```python
from build123d import *

# Parameters (mm, degrees)
SKETCH_R  = 0.95
PAD_DEPTH = 3


with BuildPart() as part:
    # Sketch → Pad (new body)
    with BuildSketch(Plane.XY):
        with BuildLine():
            ThreePointArc((1.04259, -1.342761), (1.608212, 0.551048), (0, 1.7))
            ThreePointArc((-0.965474, 1.868515), (-0.490035, 1.742445), (0, 1.7))
            Line((-5.775897, 3.600518), (-0.965474, 1.868515))
            ThreePointArc((-5.2, 6.9), (-6.874682, 5.492302), (-5.775897, 3.600518))
            Line((5.2, 6.9), (-5.2, 6.9))
            ThreePointArc((6.9, 5.2), (6.402082, 6.402082), (5.2, 6.9))
            Line((6.9, 0.351015), (6.9, 5.2))
            ThreePointArc((5.345348, -1.342761), (6.452416, -0.798531), (6.9, 0.351015))
            Line((1.182348, -1.7), (5.345348, -1.342761))
            ThreePointArc((1.04259, -1.342761), (0.978994, -1.573598), (1.182348, -1.7))
        make_face()
        with Locations((0, 5.5)):
            Circle(SKETCH_R, mode=Mode.SUBTRACT)
    extrude(amount=PAD_DEPTH)


solid = part.part
```
CAD build for the part. Positions are in the model's coordinates, mm. Coordinates: 2 decimals unless noted, no trailing zeros. Order: outer loops, then holes, each group sorted by start corner. A loop starts at its lowest first (then second) coordinate and runs counter-clockwise, first axis right, second up. Notation, with made-up numbers: (9, 36.5) - (47, 36.5) arc R17 cw to (47, 55.5) - close; hole circle Ø6 at (9, -29.75). An arc over 180 degrees is marked (long way). Answer in a Markdown table with one row per item.
1. Slice it at A-A, the plane x = 1.5. List the corners of the cut face in (y, z), then the cut area to 3 significant figures.
Answer:
| item | result |
|---|---|
| outline | (-1.67, 0) - (-0.8, 0) - (-0.8, 3) - (-1.67, 3) - close; (0.8, 0) - (6.9, 0) - (6.9, 3) - (0.8, 3) - close |
| area | 20.9 mm² |
2. Drill centre lines: L1, parallel to X at y = 6, z = 0.4; L2, parallel to Y at x = 0.5, z = 1.15; L3, parallel to X at y = 4.5, z = 1.65. Where is each one in solid material? Low to high. Write a range as from..to.
Answer:
| item | result |
|---|---|
| L1 | -6.7..-0.81, 0.81..6.7 |
| L2 | 1.62..4.69, 6.31..6.9 |
| L3 | -6.75..6.9 |
3. Pull direction X, two halves, no side cores. Call faces 1 (the face through (-0.7, 6.14, 1.48)), 2 (the face through (-6.869, 5.525, 1.479)), 3 (the face through (6.9, 3, 1)): +X half, -X half, draft (parallel to the pull), parting line (faces both ways), or undercut.
Answer:
| item | result |
|---|---|
| face 1 | undercut |
| face 2 | -X half |
| face 3 | +X half |
4. Slice it at D-D, the plane x = 5.75. List the corners of the cut face in (y, z), then the cut area to 3 significant figures.
Answer:
| item | result |
|---|---|
| outline | (-1.26, 0) - (6.81, 0) - (6.81, 3) - (-1.26, 3) - close |
| area | 24.2 mm² |
5. Slice it at C-C, the plane z = 0.45. List the corners of the cut face in (x, y), then the cut area to 3 significant figures.
Answer:
| item | result |
|---|---|
| outline | (-5.78, 3.6) - (-0.97, 1.87) arc R2.85 ccw to (0, 1.7) arc R1.7 cw to (1.04, -1.34) arc R0.2 ccw to (1.18, -1.7) - (5.35, -1.34) arc R1.7 ccw to (6.9, 0.35) - (6.9, 5.2) arc R1.7 ccw to (5.2, 6.9) - (-5.2, 6.9) arc R1.7 ccw to start; hole circle Ø1.9 at (0, 5.5) |
| area | 76.9 mm² |
6. Slice it at B-B, the plane y = 5.5. List the corners of the cut face in (x, z), then the cut area to 3 significant figures.
Answer:
| item | result |
|---|---|
| outline | (-6.87, 0) - (-0.95, 0) - (-0.95, 3) - (-6.87, 3) - close; (0.95, 0) - (6.87, 0) - (6.87, 3) - (0.95, 3) - close |
| area | 35.5 mm² |
